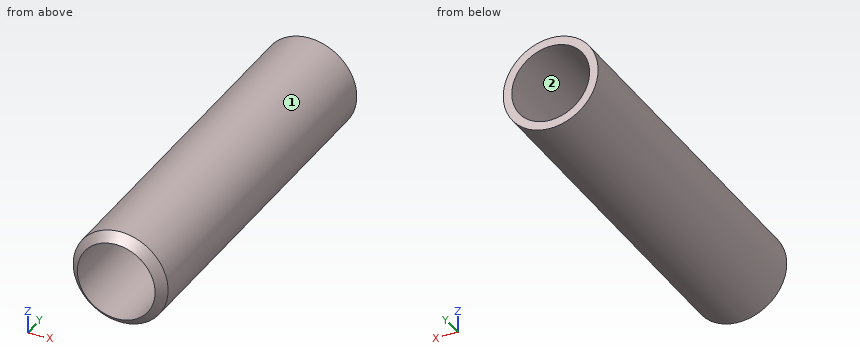
```python
from build123d import *

# Parameters (mm, degrees)
SKETCH_1_R          = 2.5
EXTRUDE_1_DEPTH     = 20
SKETCH_2_R          = 2.05
CUT_EXTRUDE_1_DEPTH = 21.310096012
CHAMFER_1_SIZE      = 1


with BuildPart() as part:
    # 草图1 → 凸台-拉伸1 (new body)
    with BuildSketch(Plane(origin=(0, 0, 0), x_dir=(1, 0, 0), z_dir=(0, 1, 0))):
        with Locations(Location((0, 0, 0), (0, 0, 270))):
            Circle(SKETCH_1_R)
    extrude(amount=EXTRUDE_1_DEPTH)

    # 草图2 → 切除-拉伸1 (cut, through all)
    with BuildSketch(Plane.XZ):
        with Locations(Location((0, 0, 0), (0, 0, 270))):
            Circle(SKETCH_2_R)
    extrude(amount=-CUT_EXTRUDE_1_DEPTH, mode=Mode.SUBTRACT)

    # 倒角1
    # the kernel refuses this chamfer: 1 mm, written as the material it takes off along each edge
    with BuildSketch(Plane(origin=(0, 0, 0), x_dir=(0, 0, 1), z_dir=(-1, 0, 0))) as chamfer_1_piece_1:
        Polygon((2.5, CHAMFER_1_SIZE), (2.5 - CHAMFER_1_SIZE, 0), (2.5, 0), align=None)
    revolve(axis=Axis((0, 0, 0), (0, 1, 0)), mode=Mode.SUBTRACT)


solid = part.part
```
CAD build for the part. Positions are in the model's coordinates, mm. Face numbers are marked on the shaded views. Coordinates: 2 decimals unless noted, no trailing zeros. Order: outer loops, then holes, each group sorted by start corner. A loop starts at its lowest first (then second) coordinate and runs counter-clockwise, first axis right, second up. Notation, with made-up numbers: (68, 21.5) - (114, 21.5) arc R28 ccw to (114, 59.5) - close; hole circle Ø4 at (14.5, 39). An arc over 180 degrees is marked (long way). Answer in a Markdown table with one row per item.
1. Flat gauge pins, fed straight in: P1, Ø1, axis at x = 1, y = 7, coming from the +Z side; P2, Ø2, axis at y = 15, z = 2, coming from the -X side. Where does each tip first touch, or does it go through?
Answer:
| item | result |
|---|---|
| P1 | z = 2.45 |
| P2 | x = -2.29 |
2. Drill centre lines: L1, parallel to Z at x = 0.1, y = 12; L2, parallel to Z at x = 0.8, y = 14.25. Where is each one in solid material? Low to high. Write a range as from..to.
Answer:
| item | result |
|---|---|
| L1 | -2.5..-2.05, 2.05..2.5 |
| L2 | -2.37..-1.89, 1.89..2.37 |
3. Slice it at C-C, the plane y = 10. List the corners of the cut face in (x, z), then the cut area to 3 significant figures.
Answer:
| item | result |
|---|---|
| outline | circle Ø5 at (0, 0); hole circle Ø4.1 at (0, 0) |
| area | 6.43 mm² |
4. Pull direction X, two halves, no side cores. Call the marked faces 1 and 2: +X half, -X half, draft (parallel to the pull), parting line (faces both ways), or undercut.
Answer:
| item | result |
|---|---|
| face 1 | parting line |
| face 2 | undercut |
5. Slice it at B-B, the plane x = 0. List the corners of the cut face in (y, z), then the cut area to 3 significant figures.
Answer:
| item | result |
|---|---|
| outline | (0.55, -2.05) - (1, -2.5) - (20, -2.5) - (20, -2.05) - close; (0.55, 2.05) - (20, 2.05) - (20, 2.5) - (1, 2.5) - close |
| area | 17.3 mm² |
6. Slice it at A-A, the plane z = 0. List the corners of the cut face in (x, y), then the cut area to 3 significant figures.
Answer:
| item | result |
|---|---|
| outline | (-2.5, 1) - (-2.05, 0.55) - (-2.05, 20) - (-2.5, 20) - close; (2.05, 0.55) - (2.5, 1) - (2.5, 20) - (2.05, 20) - close |
| area | 17.3 mm² |
